Autodesk Inventor part; units mm, degrees
ref_plane "YZ Plane" through (0, 0, 0) normal (1, 0, 0) x (0, 1, 0)
ref_plane "XZ Plane" through (0, 0, 0) normal (0, 1, 0) x (-1, 0, 0)
ref_plane "XY Plane" through (0, 0, 0) normal (0, 0, 1) x (1, 0, 0)
sketch "スケッチ1" plane through (0, 0, 0) normal (0, 0, 1) x (1, 0, 0)
  line L0 (-29.25, 22.5) -> (29.25, 22.5)
  line L1 (29.25, 22.5) -> (29.25, -22.5)
  line L2 (29.25, -22.5) -> (-29.25, -22.5)
  line L3 (-29.25, -22.5) -> (-29.25, 22.5)
  line L4 (-24.25, 19.5) -> (24.25, 19.5) construction
  line L5 (24.25, 19.5) -> (24.25, -19.5) construction
  line L6 (24.25, -19.5) -> (-24.25, -19.5) construction
  line L7 (-24.25, -19.5) -> (-24.25, 19.5) construction
  line L8 (24.25, 19.5) -> (-24.25, -19.5) construction
  line L9 (-24.25, -17.5752) -> (-24.25, 19.5)
  line L10 (-24.25, 19.5) -> (21.8563, 19.5)
  line L11 (21.8563, 19.5) -> (-24.25, -17.5752)
  line L12 (-21.8563, -19.5) -> (24.25, -19.5)
  line L13 (24.25, -19.5) -> (24.25, 17.5752)
  line L14 (24.25, 17.5752) -> (-21.8563, -19.5)
  line L15 (-29.25, 20) -> (29.25, 20) construction
  line L16 (29.25, -20) -> (-29.25, -20) construction
  line L17 (29.25, 20) -> (29.25, -20) construction
  point P0 (0, 0)
  point P1 (0, 19.5)
  point P2 (0, 22.5)
  point P3 (24.25, 0)
  point P4 (29.25, 0)
  dimension "d0" = 5
  dimension "d1" = 3
  dimension "d2" = 1.5
  dimension "d3" = 40
  dimension "d4" = 2.5
  dimension "d19" = 58.5
extrude "押し出し1" add sketch "スケッチ1" along normal blind 5
sketch "スケッチ2" plane through (29.25, -22.5, 0) normal (1, 0, 0) x (0, 0, -1)
  line L0 (0, 45) -> (-5, 45)
  line L1 (-5, 0) -> (-5, 45)
  line L2 (0, 22.5) -> (-5, 22.5) construction
  point P0 (-2.5, 2.5)
  point P1 (-2.5, 22.5)
  point P2 (-2.5, 42.5)
  point P3 (-2.5, 45)
  dimension "d7" = 40
hole "穴1" at (29.25, -20, 2.5) at (29.25, 0, 2.5) at (29.25, 20, 2.5) direction (-1, 0, 0) diameter 2.459 depth 3
mirror "ミラー1" about plane through (0, 0, 0) normal (1, 0, 0) of "穴1"
fillet "フィレット1" radius 2 6 edges at (-21.8563, -19.5, 2.5) (-24.25, -17.5752, 2.5) (24.25, 17.5752, 2.5) (24.25, -19.5, 2.5) (-24.25, 19.5, 2.5) (21.8563, 19.5, 2.5)
equation "\"d3\" = d11_1"
properties part number "リンク_ふくらはぎ_サブフレーム_1_1(予備案)" material "アルミニウム 2014-T4"
Source: CAD feature listing. Evaluate the final solid. Frame: model axes, mm. A direction names the side the tool comes from. Give positions to 0.01 mm unless a question says otherwise; leave off trailing zeros. Write each loop counter-clockwise with the first axis right and the second up, starting at its lowest first coordinate (ties: lowest second). Pieces come first, ordered by that corner, then holes.
1. First-contact query: pin 1 (0.7 mm diameter, centred on y = -19.5, z = 2.5, fed in from +X); pin 2 (3 mm diameter, centred on y = 20, z = 2.5, fed in from -X); pin 3 (5 mm diameter, centred on x = -18.5, y = -9, fed in from -Z). Flat tips, straight axial feed; report the tip coordinate or a pass-through.
2. Section query A-A (x = -1). Return the cut outline in (y, z).
3. Section query D-D (y = -4.5). Return the cut outline in (x, z).
4. Section query B-B (y = 0). Return the cut outline in (x, z), then the cut area to 3 significant figures.
5. Section query C-C (z = 2.5). Count the separate pieces of the cut face and the enclosed holes in it, then the cut area to 3 significant figures.
6. Access query for faces 1 (the face through (-1.51, 0.71, 2.46)), 2 (the face through (27.729, -0.369, 1.327)), 3 (the face through (-27.73, -21.2, 2.77)). Directions: +Z, -Z, +X, -X, +Y, -Y. A direction counts if a zero-diameter tool reaches every point of the face in a straight line with its end or side. Return the directions, or none.
7. Material intervals for line 1 along Y through (x, z) = (-28.35, 2.5); line 2 along Z through (x, y) = (27.3, -20); line 3 along X through (y, z) = (10.5, 2.65), sorted ascending.
8. Pull-direction query (Y, two-part tool) for faces 4 (the face through (-29.25, 0, 1)), 5 (the face through (-27.729, 0.369, 1.327)), 6 (the face through (0, 22.5, 2)); classes: +Y half, -Y half, draft (parallel to the pull), parting line (faces both ways), or undercut.
Output values:
1. pin 1: stops at x = 26.25
1. pin 2: stops at x = -29.25
1. pin 3: passes through
2. outline: (-22.5, 0) - (-19.5, 0) - (-19.5, 5) - (-22.5, 5) - close; (-2.73, 0) - (1.12, 0) - (1.12, 5) - (-2.73, 5) - close; (19.5, 0) - (22.5, 0) - (22.5, 5) - (19.5, 5) - close
3. outline: (-29.25, 0) - (-24.25, 0) - (-24.25, 5) - (-29.25, 5) - close; (-7.99, 0) - (-3.2, 0) - (-3.2, 5) - (-7.99, 5) - close; (24.25, 0) - (29.25, 0) - (29.25, 5) - (24.25, 5) - close
4. outline: (-29.25, 0) - (-24.25, 0) - (-24.25, 5) - (-29.25, 5) - (-29.25, 3.73) - (-26.25, 3.73) - (-26.25, 1.27) - (-29.25, 1.27) - close; (-2.39, 0) - (2.39, 0) - (2.39, 5) - (-2.39, 5) - close; (24.25, 0) - (29.25, 0) - (29.25, 1.27) - (26.25, 1.27) - (26.25, 3.73) - (29.25, 3.73) - (29.25, 5) - (24.25, 5) - close
4. area: 59.2 mm2
5. separate pieces: 1
5. enclosed holes: 2
5. area: 901 mm2
6. face 1: +Z, -Z
6. face 2: +X
6. face 3: -X
7. line 1: y = -22.5 to -21.23, -18.77 to -1.23, 1.23 to 18.77, 21.23 to 22.5
7. line 2: z = 0 to 1.27, 3.73 to 5
7. line 3: x = -29.25 to -24.25, 10.66 to 15.45, 24.25 to 29.25
8. face 4: draft
8. face 5: undercut
8. face 6: +Y half
